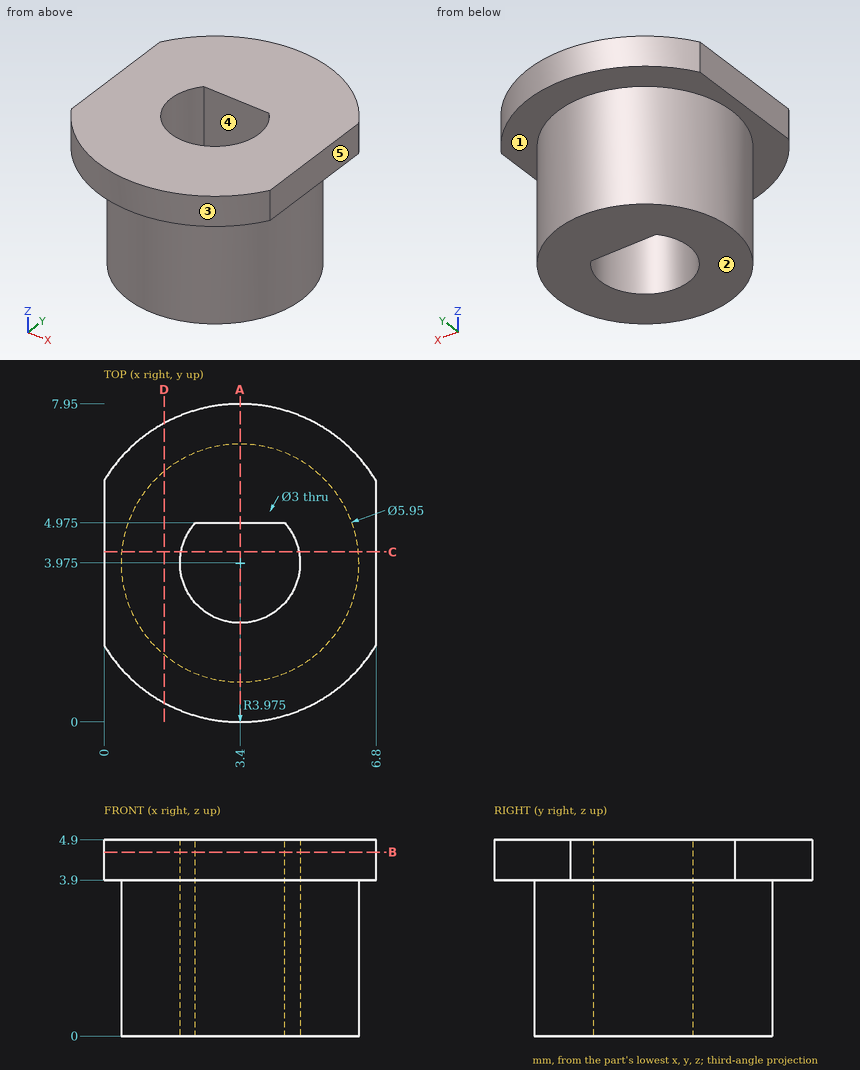
Source: three-view drawing plus pictorial views. Frame: mm from the lowest corner of the part. A direction names the side the tool comes from. Round coordinates to 2 decimals unless told otherwise and drop trailing zeros. Write each loop counter-clockwise with the first axis right and the second up, starting at its lowest first coordinate (ties: lowest second). Pieces come first, ordered by that corner, then holes. Notation, with made-up numbers: M 21.5,24.25 L 50.5,24.25 A33 cw 50.5,55.25 Z; hole C 86,-6.75 d8. An arc over 180 degrees is marked long. Write item = value, one per line.
Item 1: Section query D-D on x = 1.5. Return loops of the section in (y, z), then the cut area to 3 significant figures.
Findings:
outline = M 0.48,3.9 L 1.69,3.9 L 1.69,0 L 6.26,0 L 6.26,3.9 L 7.47,3.9 L 7.47,4.9 L 0.48,4.9 Z
area = 24.8 mm^2
Item 2: Pull-direction query (Y, two-part tool) for the marked faces 3, 4 and 5; classes: pulls with the +Y half, pulls with the -Y half, needs draft (parallel to the pull), parting line crosses it, or undercut.
Findings:
face_3 = pulls with the -Y half
face_4 = undercut
face_5 = needs draft
Item 3: Access query for the marked faces 1 and 2. Directions: +Z, -Z, +X, -X, +Y, -Y. A direction counts if a zero-diameter tool reaches every point of the face in a straight line with its end or side. Return the directions, or none.
Findings:
face_1 = -Z
face_2 = -Z, +X, -X, +Y, -Y
Item 4: Section query B-B on z = 4.6. Return loops of the section in (x, y) (3 decimals).
Findings:
outline = M 0,1.916 A3.975 ccw 6.8,1.916 L 6.8,6.034 A3.975 ccw 0,6.034 Z; hole M 2.282,4.975 A1.5 ccw long 4.518,4.975 Z
Item 5: Material intervals for line 1 along Z through (x, y) = (0.5, 1.5); line 2 along Y through (x, z) = (4.5, 4) (3 decimals); line 3 along Y through (x, z) = (2.5, 3.8) (3 decimals), sorted ascending. Write a range as [from, to].
Findings:
line_1 = [3.9, 4.9]
line_2 = [0.155, 2.955], [4.975, 7.795]
line_3 = [1.139, 2.775], [4.975, 6.811]
Item 6: Pin query (flat end, axial travel): P1, Ø1.8, axis at x = 3, z = 2, coming from the -Y side; P2, Ø1.5, axis at y = 1, z = 0.5, coming from the +X side; P3, Ø2, axis at y = 6, z = 0.5, coming from the -X side; P4, Ø2.5, axis at x = 3.4, y = 3.975, coming from the +Z side. Return the tip coordinate at first contact, or that it passes through.
Findings:
P1 = 1
P2 = 5.37
P3 = 0.61
P4 = 4.9
Item 7: Section query C-C on y = 4.25. Return loops of the section in (x, z), then the cut area to 3 significant figures.
Findings:
outline = M 0,3.9 L 0.44,3.9 L 0.44,0 L 1.93,0 L 1.93,4.9 L 0,4.9 Z; M 4.87,0 L 6.36,0 L 6.36,3.9 L 6.8,3.9 L 6.8,4.9 L 4.87,4.9 Z
area = 15.5 mm^2
Item 8: Section query A-A on x = 3.4. Return loops of the section in (y, z) (3 decimals).
Findings:
outline = M 0,3.9 L 1,3.9 L 1,0 L 2.475,0 L 2.475,4.9 L 0,4.9 Z; M 4.975,0 L 6.95,0 L 6.95,3.9 L 7.95,3.9 L 7.95,4.9 L 4.975,4.9 Z
